```python
from build123d import *

# Parameters (mm, degrees)
CROQUIS1_W              = 170
CROQUIS1_H              = 50
SALIENTE_EXTRUIR1_DEPTH = 4
SALIENTE_EXTRUIR2_DEPTH = 70
SALIENTE_EXTRUIR3_DEPTH = 25
SALIENTE_EXTRUIR4_DEPTH = 64
SALIENTE_EXTRUIR5_DEPTH = 25
CROQUIS9_W              = 17
CROQUIS9_H              = 17.5
CROQUIS9_W_2            = 56
CORTAR_EXTRUIR1_DEPTH   = 70
CROQUIS11_W             = 64
CROQUIS11_H             = 55
CORTAR_EXTRUIR4_DEPTH   = 15
CROQUIS12_R             = 1.75
CORTAR_EXTRUIR5_DEPTH   = 15
CORTAR_EXTRUIR6_DEPTH   = 1


with BuildPart() as part:
    # Croquis1 → Saliente-Extruir1 (new body)
    with BuildSketch(Plane.XY):
        Rectangle(CROQUIS1_W, CROQUIS1_H)
    extrude(amount=SALIENTE_EXTRUIR1_DEPTH)

    # Croquis3 → Saliente-Extruir2 (add)
    with BuildSketch(Plane.XY.offset(4)):
        Polygon((-85, 7.5), (85, 7.5), (85, -7.5), (60, -7.5), (60, -11.921199344), (56, -11.921199344), (54.5, -11.921199344), (54.5, -8.921199344), (56, -8.921199344), (56, -2.921199344), (36, -2.921199344), (36, -8.921199344), (37.5, -8.921199344), (37.5, -11.921199344), (36, -11.921199344), (32, -11.921199344), (32, -7.5), (-32, -7.5), (-32, -11.921199344), (-36, -11.921199344), (-37.5, -11.921199344), (-37.5, -8.921199344), (-36, -8.921199344), (-36, -2.921199344), (-56, -2.921199344), (-56, -8.921199344), (-54.5, -8.921199344), (-54.5, -11.921199344), (-56, -11.921199344), (-60, -11.921199344), (-60, -7.5), (-85, -7.5), align=None)
    extrude(amount=SALIENTE_EXTRUIR2_DEPTH)

    # Croquis4 → Saliente-Extruir3 (add)
    with BuildSketch(Plane.ZY.offset(85)):
        Polygon((4, -25), (19, -7.5), (4, -7.5), align=None)
    saliente_extruir3 = extrude(amount=-SALIENTE_EXTRUIR3_DEPTH)

    # Croquis5 → Saliente-Extruir4 (add)
    with BuildSketch(Plane.ZY.offset(-32)):
        Polygon((19, -7.5), (4, -25), (4, -7.5), align=None)
    saliente_extruir4 = extrude(amount=SALIENTE_EXTRUIR4_DEPTH)

    # Croquis7 → Saliente-Extruir5 (add)
    with BuildSketch(Plane(origin=(60, 0, 0), x_dir=(0, 0, -1), z_dir=(1, 0, 0))):
        Polygon((-4, -25), (-19, -7.5), (-4, -7.5), align=None)
    saliente_extruir5 = extrude(amount=SALIENTE_EXTRUIR5_DEPTH)

    # Croquis9 → Cortar-Extruir1 (cut)
    with BuildSketch(Plane.XY.offset(74)):
        with Locations((-72.5, -16.25)):
            Rectangle(CROQUIS9_W, CROQUIS9_H)
        with Locations((0, -16.25)):
            Rectangle(CROQUIS9_W_2, CROQUIS9_H)
        with Locations((72.5, -16.25)):
            Rectangle(CROQUIS9_W, CROQUIS9_H)
    cortar_extruir1 = extrude(amount=-CORTAR_EXTRUIR1_DEPTH, mode=Mode.SUBTRACT)

    # Croquis11 → Cortar-Extruir4 (cut)
    with BuildSketch(Plane.XZ.offset(7.5)):
        with Locations((0, 46.5)):
            Rectangle(CROQUIS11_W, CROQUIS11_H)
    extrude(amount=-CORTAR_EXTRUIR4_DEPTH, mode=Mode.SUBTRACT)

    # Croquis12 → Cortar-Extruir5 (cut)
    with BuildSketch(Plane.XY.offset(4)):
        with Locations((-72.5, 15.138462845)):
            Circle(CROQUIS12_R)
        with Locations((-72.5, -15.138462845)):
            Circle(CROQUIS12_R)
        with Locations((72.5, -15.138462845)):
            Circle(CROQUIS12_R)
        with Locations((72.5, 15.138462845)):
            Circle(CROQUIS12_R)
    extrude(amount=-CORTAR_EXTRUIR5_DEPTH, mode=Mode.SUBTRACT)

    # Croquis14 → Cortar-Extruir6 (cut)
    with BuildSketch(Plane.ZY.offset(85)):
        Polygon((19, -7.5), (4, -7.5), (4, -25), align=None)
    cortar_extruir6 = extrude(amount=-CORTAR_EXTRUIR6_DEPTH, mode=Mode.SUBTRACT)

    # Simetría1: Saliente-Extruir3, Saliente-Extruir4, Saliente-Extruir5, Cortar-Extruir1, Cortar-Extruir6 across plane
    add(saliente_extruir3.mirror(Plane(origin=(0, 0, 0), x_dir=(0, 0, 1), z_dir=(0, -1, 0))))
    add(saliente_extruir4.mirror(Plane(origin=(0, 0, 0), x_dir=(0, 0, 1), z_dir=(0, -1, 0))))
    add(saliente_extruir5.mirror(Plane(origin=(0, 0, 0), x_dir=(0, 0, 1), z_dir=(0, -1, 0))))
    add(cortar_extruir1.mirror(Plane(origin=(0, 0, 0), x_dir=(0, 0, 1), z_dir=(0, -1, 0))), mode=Mode.SUBTRACT)
    add(cortar_extruir6.mirror(Plane(origin=(0, 0, 0), x_dir=(0, 0, 1), z_dir=(0, -1, 0))), mode=Mode.SUBTRACT)


solid = part.part
```
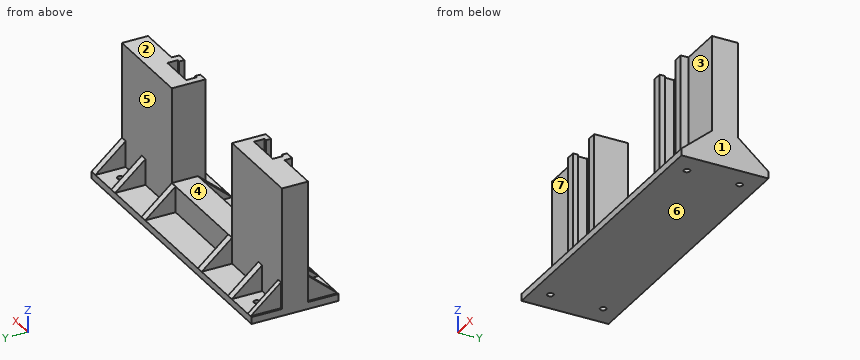
Geometry: final body of the model. Coordinates: model frame, mm. Face numbers are marked on the shaded views. A direction names the side the tool comes from. Give positions to 0.01 mm unless a question says otherwise; leave off trailing zeros. Write each loop counter-clockwise with the first axis right and the second up, starting at its lowest first coordinate (ties: lowest second). Pieces come first, ordered by that corner, then holes.
1. Line query: probe 1 along Y at (x, z) = (-72.5, 1.55); probe 2 along X at (y, z) = (9, 12); probe 3 along X at (y, z) = (-3, 60). Output: solid intervals per line, ascending.
2. Reachability of the marked faces 4, 5, 6 and 7 from +Z, -Z, +X, -X, +Y, -Y: full face, straight path, thin tool, end or side. Return the list, or none.
3. Section query A-A, the plane x = -72.5. Return loops of the section in (y, z), then the cut area to 3 significant figures.
4. Section query D-D, the plane x = -22. Return loops of the section in (y, z).
5. Section query C-C, the plane x = 68.5. Return loops of the section in (y, z).
6. Section query B-B, the plane z = 41. Return loops of the section in (x, y), then the cut area to 3 significant figures.
7. Draft query along X for the marked faces 1, 2 and 3. Return one class per face: released by +X, released by -X, zero draft, split by the parting line, or undercut.
8. Pin query (flat end, axial travel): P1, Ø6, axis at x = -9.5, y = -14.5, coming from the +Z side; P2, Ø0.8, axis at x = 55.5, z = 27, coming from the +Y side; P3, Ø4.5, axis at y = 14.5, z = 13.5, coming from the -X side. Return the tip coordinate at first contact, or that it passes through.
Computed:
1. probe 1: y = -25 to -16.89, -13.39 to 13.39, 16.89 to 25
1. probe 2: x = -84 to -81, -64 to -60, -32 to -28, 28 to 32, 60 to 64, 81 to 85
1. probe 3: x = -85 to -56, -36 to -32, 32 to 36, 56 to 85
2. face 4: +Z, +Y, -Y
2. face 5: +Z, +Y
2. face 6: -Z, +X, -X, +Y, -Y
2. face 7: +Z, -Y
3. outline: (-25, 0) - (-16.89, 0) - (-16.89, 4) - (-25, 4) - close; (-13.39, 0) - (13.39, 0) - (13.39, 4) - (7.5, 4) - (7.5, 74) - (-7.5, 74) - (-7.5, 4) - (-13.39, 4) - close; (16.89, 0) - (25, 0) - (25, 4) - (16.89, 4) - close
3. area: 1,220 mm2
4. outline: (-25, 0) - (25, 0) - (25, 4) - (7.5, 4) - (7.5, 19) - (-7.5, 19) - (-7.5, 4) - (-25, 4) - close
5. outline: (-25, 0) - (25, 0) - (25, 4) - (7.5, 4) - (7.5, 74) - (-7.5, 74) - (-7.5, 4) - (-25, 4) - close
6. outline: (-85, -7.5) - (-60, -7.5) - (-60, -11.92) - (-54.5, -11.92) - (-54.5, -8.92) - (-56, -8.92) - (-56, -2.92) - (-36, -2.92) - (-36, -8.92) - (-37.5, -8.92) - (-37.5, -11.92) - (-32, -11.92) - (-32, 7.5) - (-85, 7.5) - close; (32, -11.92) - (37.5, -11.92) - (37.5, -8.92) - (36, -8.92) - (36, -2.92) - (56, -2.92) - (56, -8.92) - (54.5, -8.92) - (54.5, -11.92) - (60, -11.92) - (60, -7.5) - (85, -7.5) - (85, 7.5) - (32, 7.5) - close
6. area: 1,500 mm2
7. face 1: released by +X
7. face 2: zero draft
7. face 3: undercut
8. P1: stops at z = 4
8. P2: stops at y = 7.5
8. P3: stops at x = -84
